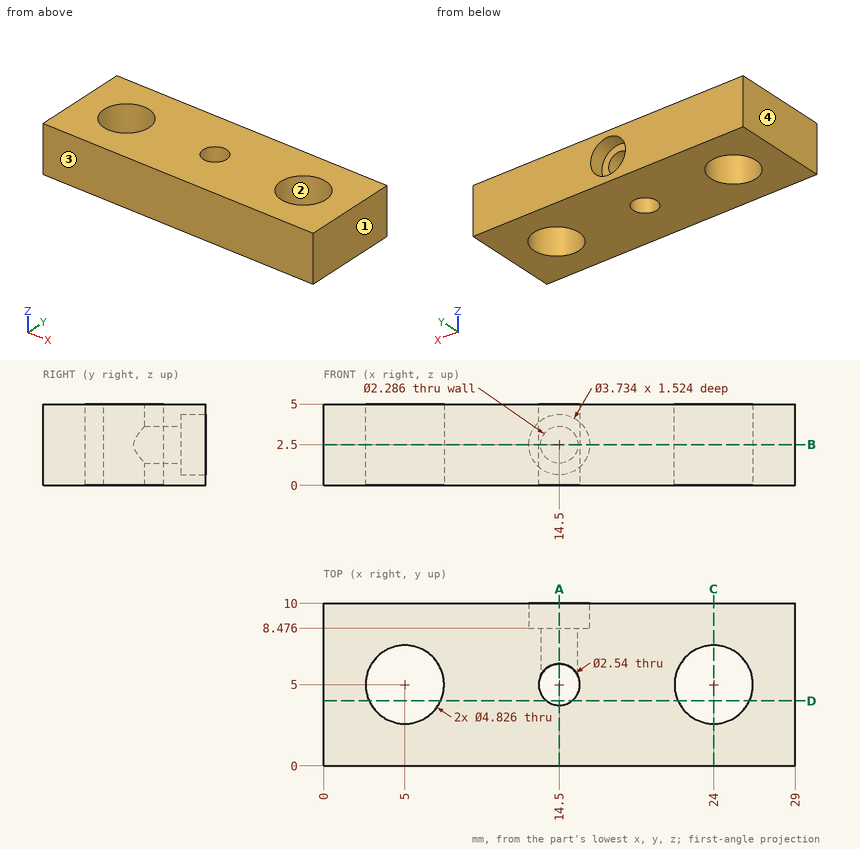
Here's the drawing with two shaded views (mm, measured from the low corner). I have some questions. Round coordinates to 2 decimals unless told otherwise and drop trailing zeros. Write each loop counter-clockwise with the first axis right and the second up, starting at its lowest first coordinate (ties: lowest second). Pieces come first, ordered by that corner, then holes. Notation, with made-up numbers: M 5.25,88.5 L 61.25,88.5 A30 ccw 61.25,124.5 Z; hole C -30.5,-21.5 d5. An arc over 180 degrees is marked long. Answer in a Markdown table with one row per item. Add a question column.
Q1. If we mould it in two halves opening along X, with no side actions, what happens to the marked faces 1, 2, 3 and 4? For each: +X half, -X half, draft (parallel to the pull), parting line (faces both ways), or undercut.
Q2. Imagine slicing it at D-D (y = 4). Please give me the cut outline in (x, z).
Q3. If I drill on line 1 (Z direction, x = 14.5, y = 6.3); line 2 (Z direction, x = 14.5, y = 9.2); line 3 (Y direction, x = 24, z = 2.6), over which ranges is the centre line in solid material (lowest first)? Write a range as from..to.
Q4. Imagine slicing it at B-B (z = 2.5). Please give me the cut outline in (x, y), then the cut area to 3 significant figures.
Q5. Will this pin go through, and if not, where does the flat tip stop? pin 1 Ø1.1 at (x, z) = (14, 2) entering from +Y.
Q6. Imagine slicing it at C-C (x = 24). Please give me the cut outline in (y, z).
Q7. Imagine slicing it at A-A (x = 14.5). Please give me the cut outline in (y, z), then the cut area to 3 significant figures.
Values:
| question | item | result |
|---|---|---|
| 1 | face 1 | +X half |
| 1 | face 2 | undercut |
| 1 | face 3 | draft |
| 1 | face 4 | -X half |
| 2 | outline | M 0,0 L 2.8,0 L 2.8,5 L 0,5 Z; M 7.2,0 L 13.72,0 L 13.72,5 L 7.2,5 Z; M 15.28,0 L 21.8,0 L 21.8,5 L 15.28,5 Z; M 26.2,0 L 29,0 L 29,5 L 26.2,5 Z |
| 3 | line 1 | 0..1.36, 3.64..5 |
| 3 | line 2 | 0..0.63, 4.37..5 |
| 3 | line 3 | 0..2.59, 7.41..10 |
| 4 | outline | M 0,0 L 29,0 L 29,10 L 16.37,10 L 16.37,8.48 L 15.64,8.48 L 15.64,5.55 A1.27 cw long 13.36,5.55 L 13.36,8.48 L 12.63,8.48 L 12.63,10 L 0,10 Z; hole C 5,5 d4.83; hole C 24,5 d4.83 |
| 4 | area | 237 mm^2 |
| 5 | pin 1 | y = 8.48 |
| 6 | outline | M 0,0 L 2.59,0 L 2.59,5 L 0,5 Z; M 7.41,0 L 10,0 L 10,5 L 7.41,5 Z |
| 7 | outline | M 0,0 L 3.73,0 L 3.73,5 L 0,5 Z; M 6.27,0 L 10,0 L 10,0.63 L 8.48,0.63 L 8.48,1.36 L 6.27,1.36 Z; M 6.27,3.64 L 8.48,3.64 L 8.48,4.37 L 10,4.37 L 10,5 L 6.27,5 Z |
| 7 | area | 26.6 mm^2 |
